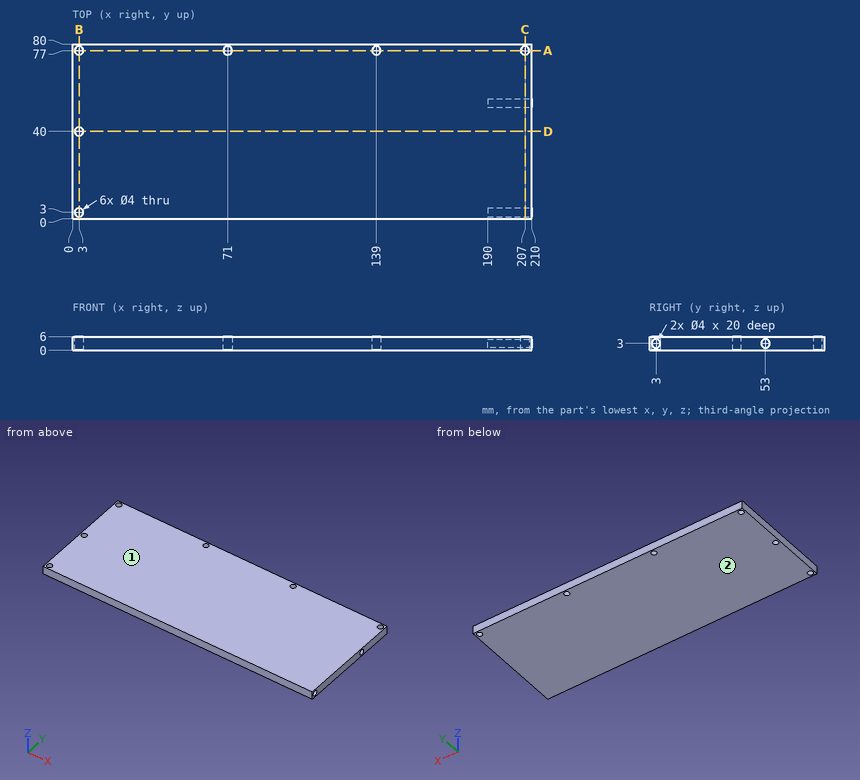
Part print with two shaded views. Sizes in mm from the minimum x, y, z corner. Round coordinates to 2 decimals unless told otherwise and drop trailing zeros. Order: outer loops, then holes, each group sorted by start corner. A loop starts at its lowest first (then second) coordinate and runs counter-clockwise, first axis right, second up. Notation, with made-up numbers: M 47.5,1 L 63.5,1 A8 ccw 63.5,15 Z; hole C 65.25,-1.5 d4. An arc over 180 degrees is marked long. Answer in a Markdown table with one row per item. Add a question column.
Q1. Cut at B-B on x = 3. Give the cut face in (y, z), and give its area (3 significant figures).
Q2. Cut at C-C on x = 207. Give the cut face in (y, z).
Q3. Pin check, flat tips, straight feed: pin 1 (3.5 mm diameter, centred on x = 3, y = 40, fed in from +Z); pin 2 (2.5 mm diameter, centred on y = 3, z = 3, fed in from +X). Stop position of each tip, or through.
Q4. Cut at D-D on y = 40. Give the cut face in (x, z), and give its area (3 significant figures).
Q5. Mould opens along Z. For the marked faces 1 and 2 say: +Z half, -Z half, draft (parallel to the pull), parting line (faces both ways), or undercut.
Q6. Wall check: L1, parallel to Y at x = 203.75, z = 3; L2, parallel to X at y = 77, z = 2.05; L3, parallel to Y at x = 3, z = 2.95. Give the ranges that are in metal, low to high. Write a range as from..to.
Q7. Cut at A-A on y = 77. Give the cut face in (x, z).
Established:
| question | item | result |
|---|---|---|
| 1 | outline | M 0,0 L 1,0 L 1,6 L 0,6 Z; M 5,0 L 38,0 L 38,6 L 5,6 Z; M 42,0 L 75,0 L 75,6 L 42,6 Z; M 79,0 L 80,0 L 80,6 L 79,6 Z |
| 1 | area | 408 mm2 |
| 2 | outline | M 0,0 L 75,0 L 75,6 L 0,6 Z; M 79,0 L 80,0 L 80,6 L 79,6 Z; hole C 3,3 d4; hole C 53,3 d4 |
| 3 | pin 1 | passes through |
| 3 | pin 2 | stops at x = 190 |
| 4 | outline | M 0,0 L 1,0 L 1,6 L 0,6 Z; M 5,0 L 210,0 L 210,6 L 5,6 Z |
| 4 | area | 1,240 mm2 |
| 5 | face 1 | +Z half |
| 5 | face 2 | -Z half |
| 6 | L1 | y = 0..1, 5..51, 55..80 |
| 6 | L2 | x = 0..1, 5..69, 73..137, 141..205, 209..210 |
| 6 | L3 | y = 0..1, 5..38, 42..75, 79..80 |
| 7 | outline | M 0,0 L 1,0 L 1,6 L 0,6 Z; M 5,0 L 69,0 L 69,6 L 5,6 Z; M 73,0 L 137,0 L 137,6 L 73,6 Z; M 141,0 L 205,0 L 205,6 L 141,6 Z; M 209,0 L 210,0 L 210,6 L 209,6 Z |
